Verification items for the finished model (mm, model axes). Face numbers are marked on the shaded views. Give positions to 0.01 mm unless a question says otherwise; leave off trailing zeros. Loops run counter-clockwise (first coordinate to the right, second up) from the corner with the lowest first, then second, coordinate; pieces in that order, holes last. Notation, with made-up numbers: (-19.5, 71.25) -> (1.5, 71.25) arc R22 ccw to (1.5, 78.25) -> close; hole circle Ø1 at (-23, 81.25). An arc over 180 degrees is marked (long way). Answer in a Markdown table with one row per item. Add a question column.
Q1. Section check C-C on y = 3.9. Enter the section's corners in (x, z).
Q2. Release check for a two-part mould opening along X. For the marked faces 1 and 2 record: pulls with the +X half, pulls with the -X half, needs draft (parallel to the pull), parting line crosses it, or undercut.
Q3. Section check D-D on x = 2.25. Enter the section's corners in (y, z), and give its area (3 significant figures).
Q4. Gauge pin test, flat ends, axial feed: P1, Ø1.5, axis at y = 0.5, z = 1.5, coming from the +X side; P2, Ø2.5, axis at y = 3, z = 5.5, coming from the -X side; P3, Ø1.5, axis at x = -3.5, y = 3, coming from the -Z side. Record the tip position at first contact, or that the pin passes through.
Q5. Material ranges on probe 1 along Z at (x, y) = (0, 3.1); probe 2 along X at (y, z) = (2.35, 21.75); probe 3 along Z at (x, y) = (0.75, 1.35), recorded low to high.
Q6. Section check B-B on x = 0. Enter the section's corners in (y, z).
Q7. Section check A-A on z = -21.75. Enter the section's corners in (x, y), and give its area (3 significant figures).
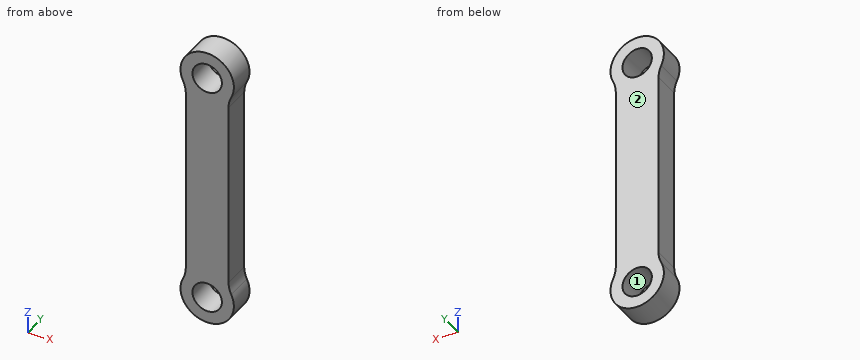
```python
from build123d import *

# Parameters (mm, degrees)
BOSS_EXTRUDE1_DEPTH = 5
SKETCH2_R           = 2.75
CUT_EXTRUDE2_DEPTH  = 6
SKETCH3_R           = 5
SKETCH3_R_2         = 2.75
BOSS_EXTRUDE2_DEPTH = 5
FILLET1_R           = 5


with BuildPart() as part:
    # Sketch1 → Boss-Extrude1 (new body)
    with BuildSketch(Plane(origin=(0, 0, 0), x_dir=(1, 0, 0), z_dir=(0, 1, 0))):
        with BuildLine():
            Line((-4, -21.75), (-4, 21.75))
            ThreePointArc((-4, 21.75), (0, 25.75), (4, 21.75))
            Line((4, 21.75), (4, -21.75))
            ThreePointArc((4, -21.75), (0, -25.75), (-4, -21.75))
        make_face()
    extrude(amount=BOSS_EXTRUDE1_DEPTH)

    # Sketch2 → Cut-Extrude2 (cut, through all)
    with BuildSketch(Plane(origin=(0, 5, 0), x_dir=(1, 0, 0), z_dir=(0, 1, 0))):
        with Locations((0, 21.75)):
            Circle(SKETCH2_R)
        with Locations((0, -21.75)):
            Circle(SKETCH2_R)
    extrude(amount=-CUT_EXTRUDE2_DEPTH, mode=Mode.SUBTRACT)

    # Sketch3 → Boss-Extrude2 (add)
    with BuildSketch(Plane(origin=(0, 5, 0), x_dir=(1, 0, 0), z_dir=(0, 1, 0))):
        with Locations((0, 21.75)):
            Circle(SKETCH3_R)
        with Locations((0, 21.75)):
            Circle(SKETCH3_R_2, mode=Mode.SUBTRACT)
        with Locations((0, -21.75)):
            Circle(SKETCH3_R)
        with Locations((0, -21.75)):
            Circle(SKETCH3_R_2, mode=Mode.SUBTRACT)
    extrude(amount=-BOSS_EXTRUDE2_DEPTH)

    # Fillet1
    fillet1_edges = [part.edges().sort_by_distance(p)[0] for p in [
        (-4, 2.5, -18.75),
        (4, 2.5, -18.75),
        (-4, 2.5, 18.75),
        (4, 2.5, 18.75),
    ]]
    fillet(fillet1_edges, radius=FILLET1_R)


solid = part.part
```
Taken from the geometry:
| question | item | result |
|---|---|---|
| 1 | outline | (-4.5, -19.57) arc R5 ccw (long way) to (4.5, -19.57) arc R5 cw to (4, -17.39) -> (4, 17.39) arc R5 cw to (4.5, 19.57) arc R5 ccw (long way) to (-4.5, 19.57) arc R5 cw to (-4, 17.39) -> (-4, -17.39) arc R5 cw to start; hole circle Ø5.5 at (0, -21.75); hole circle Ø5.5 at (0, 21.75) |
| 2 | face 1 | undercut |
| 2 | face 2 | needs draft |
| 3 | outline | (0, -26.22) -> (5, -26.22) -> (5, -23.33) -> (0, -23.33) -> close; (0, -20.17) -> (5, -20.17) -> (5, 20.17) -> (0, 20.17) -> close; (0, 23.33) -> (5, 23.33) -> (5, 26.22) -> (0, 26.22) -> close |
| 3 | area | 231 mm² |
| 4 | P1 | stops at x = 4 |
| 4 | P2 | stops at x = -4 |
| 4 | P3 | stops at z = -25.93 |
| 5 | probe 1 | z = -26.75 to -24.5, -19 to 19, 24.5 to 26.75 |
| 5 | probe 2 | x = -5 to -2.75, 2.75 to 5 |
| 5 | probe 3 | z = -26.69 to -24.4, -19.1 to 19.1, 24.4 to 26.69 |
| 6 | outline | (0, -26.75) -> (5, -26.75) -> (5, -24.5) -> (0, -24.5) -> close; (0, -19) -> (5, -19) -> (5, 19) -> (0, 19) -> close; (0, 24.5) -> (5, 24.5) -> (5, 26.75) -> (0, 26.75) -> close |
| 7 | outline | (-5, 0) -> (-2.75, 0) -> (-2.75, 5) -> (-5, 5) -> close; (2.75, 0) -> (5, 0) -> (5, 5) -> (2.75, 5) -> close |
| 7 | area | 22.5 mm² |
